Build history of the part. All positions in model axes, mm. Give positions to 0.01 mm unless a question says otherwise; leave off trailing zeros. Order: outer loops, then holes, each group sorted by start corner. A loop starts at its lowest first (then second) coordinate and runs counter-clockwise, first axis right, second up. Notation, with made-up numbers: (-31.5, -29) -> (-21.5, -29) arc R22 ccw to (-21.5, 1) -> close; hole circle Ø11 at (83, -27). An arc over 180 degrees is marked (long way). One line per item, written item: value. Start each with the question number.
(1) Probe line 1 (Z direction, x = 0, y = -0.6); line 2 (X direction, y = 0.75, z = 3); line 3 (X direction, y = 1.15, z = 0). List the from-to ranges inside material, lowest first.
(2) Pin check, flat tips, straight feed: pin 1 (1 mm diameter, centred on y = 1, z = -3.5, fed in from -X); pin 2 (2 mm diameter, centred on x = 3.5, y = 0, fed in from -Z). Stop position of each tip, or through.
(3) Saw through at A-A on y = -1.75. Give the cut face in (x, z).
```python
from build123d import *

# Parameters (mm, degrees)
SKETCH1_R           = 5
BOSS_EXTRUDE1_DEPTH = 3
CHAMFER1_SIZE       = 0.5
SKETCH2_OUTSIDE_W   = 62.08
SKETCH2_OUTSIDE_H   = 59.51
SKETCH2_OUTSIDE_R   = 8.660766964
CUT_EXTRUDE1_DEPTH  = 10
CUT_EXTRUDE1_TAPER  = 60


with BuildPart() as part:
    # Sketch1 → Boss-Extrude1 (new body, symmetric)
    with BuildSketch(Plane(origin=(0, 0, 0), x_dir=(1, 0, 0), z_dir=(0, 1, 0))):
        Polygon((-4.905742916, -8.714673391), (5.094257084, -8.605834685), (10, 0.108838706), (4.905742916, 8.714673391), (-5.094257084, 8.605834685), (-10, -0.108838706), align=None)
        Circle(SKETCH1_R, mode=Mode.SUBTRACT)
    extrude(amount=BOSS_EXTRUDE1_DEPTH, both=True)

    # Chamfer1
    chamfer1_edges = [part.edges().sort_by_distance(p)[0] for p in [
        (-5, -3, 0),
        (-5, 3, 0),
    ]]
    chamfer(chamfer1_edges, length=CHAMFER1_SIZE)

    # Sketch2 outside → Cut-Extrude1 (cut)
    with BuildSketch(Plane(origin=(0, 3, 0), x_dir=(1, 0, 0), z_dir=(0, 1, 0))):
        Rectangle(SKETCH2_OUTSIDE_W, SKETCH2_OUTSIDE_H)
        Circle(SKETCH2_OUTSIDE_R, mode=Mode.SUBTRACT)
    cut_extrude1 = extrude(amount=-CUT_EXTRUDE1_DEPTH, taper=CUT_EXTRUDE1_TAPER, mode=Mode.SUBTRACT)

    # Mirror1: Cut-Extrude1 across plane
    add(cut_extrude1.mirror(Plane.ZX), mode=Mode.SUBTRACT)


solid = part.part
```
Results below:
1. line 1: z = -8.66 to -5, 5 to 8.66
1. line 2: x = -8.29 to -4, 4 to 8.25
1. line 3: x = -9.94 to -5, 5 to 9.94
2. pin 1: stops at x = -8.25
2. pin 2: stops at z = -8.71
3. outline: (-10, 0.11) -> (-5.09, -8.61) -> (4.91, -8.71) -> (10, -0.11) -> (5.09, 8.61) -> (-4.91, 8.71) -> close; hole circle Ø10 at (0, 0)
